Build history of the part. All positions in model axes, mm. A direction names the side the tool comes from. Give positions to 0.01 mm unless a question says otherwise; leave off trailing zeros. Order: outer loops, then holes, each group sorted by start corner. A loop starts at its lowest first (then second) coordinate and runs counter-clockwise, first axis right, second up. Notation, with made-up numbers: M 24.5,54 L 77.5,54 A18 ccw 77.5,77 Z; hole C 69.5,35.25 d7. An arc over 180 degrees is marked long. One line per item, written item: value.
from build123d import *

# Parameters (mm, degrees)
SKETCH1_W           = 25
SKETCH1_H           = 38
BOSS_EXTRUDE1_DEPTH = 1.425
SKETCH2_R           = 2
CUT_EXTRUDE1_DEPTH  = 23.92100565
SKETCH3_R           = 0.8
CUT_EXTRUDE2_DEPTH  = 23.92100565
SKETCH4_W           = 5
SKETCH4_H           = 2.85
BOSS_EXTRUDE2_DEPTH = 2.85
SKETCH5_W           = 8
SKETCH5_H           = 2.9
CUT_EXTRUDE3_DEPTH  = 26.333673243
SKETCH6_W           = 3.5
SKETCH6_H           = 8.95
CUT_EXTRUDE4_DEPTH  = 26.333673243
FILLET1_R           = 5


with BuildPart() as part:
    # Sketch1 → Boss-Extrude1 (new, symmetric)
    with BuildSketch(Plane.XY):
        Rectangle(SKETCH1_W, SKETCH1_H)
    extrude(amount=BOSS_EXTRUDE1_DEPTH, both=True)

    # Sketch2 → Cut-Extrude1 (cut, through all)
    with BuildSketch(Plane.XY.offset(1.425)):
        with Locations((0, -14)):
            Circle(SKETCH2_R)
    extrude(amount=-CUT_EXTRUDE1_DEPTH, mode=Mode.SUBTRACT)

    # Sketch3 → Cut-Extrude2 (cut, through all)
    with BuildSketch(Plane.XY.offset(1.425)):
        with Locations((-4.8, -14)):
            Circle(SKETCH3_R)
        with Locations((4.8, -14)):
            Circle(SKETCH3_R)
    extrude(amount=-CUT_EXTRUDE2_DEPTH, mode=Mode.SUBTRACT)

    # Sketch4 → Boss-Extrude2 (add)
    with BuildSketch(Plane.XY.offset(1.425)):
        with Locations((-4.25, 20.425)):
            Rectangle(SKETCH4_W, SKETCH4_H)
        with Locations((4.25, 20.425)):
            Rectangle(SKETCH4_W, SKETCH4_H)
    extrude(amount=-BOSS_EXTRUDE2_DEPTH)

    # Sketch5 → Cut-Extrude3 (cut, through all)
    with BuildSketch(Plane.XY.offset(1.425)):
        with Locations((0, 14.5)):
            Rectangle(SKETCH5_W, SKETCH5_H)
    extrude(amount=-CUT_EXTRUDE3_DEPTH, mode=Mode.SUBTRACT)

    # Sketch6 → Cut-Extrude4 (cut, through all)
    with BuildSketch(Plane.XY.offset(1.425)):
        with Locations((0, 14.525)):
            Rectangle(SKETCH6_W, SKETCH6_H)
    extrude(amount=-CUT_EXTRUDE4_DEPTH, mode=Mode.SUBTRACT)

    # Fillet1
    fillet1_edges = [part.edges().sort_by_distance(p)[0] for p in [
        (12.5, -19, 0),
        (-12.5, -19, 0),
    ]]
    fillet(fillet1_edges, radius=FILLET1_R)


solid = part.part
1) Saw through at D-D, the plane x = -8.75. Write the cut outline in (y, z) (3 decimals), then the cut area to 3 significant figures.
Check values:
outline: M -18.841,-1.425 L 19,-1.425 L 19,1.425 L -18.841,1.425 Z
area: 108 mm^2
2) Saw through at B-B, the plane z = -1. Write the cut outline in (x, y), then the cut area to 3 significant figures.
Check values:
outline: M -12.5,-14 A5 ccw -7.5,-19 L 7.5,-19 A5 ccw 12.5,-14 L 12.5,19 L 6.75,19 L 6.75,21.85 L 1.75,21.85 L 1.75,15.95 L 4,15.95 L 4,13.05 L 1.75,13.05 L 1.75,10.05 L -1.75,10.05 L -1.75,13.05 L -4,13.05 L -4,15.95 L -1.75,15.95 L -1.75,21.85 L -6.75,21.85 L -6.75,19 L -12.5,19 Z; hole C -4.8,-14 d1.6; hole C 0,-14 d4; hole C 4.8,-14 d1.6
area: 907 mm^2
3) Mould opens along Y. For faces 1 (the face through (-12.5, 2, 0)), 2 (the face through (-3, 15.95, 0)), 3 (the face through (-4, 21.85, 0)) say: released by +Y, released by -Y, zero draft, split by the parting line, or undercut.
Check values:
face 1: zero draft
face 2: undercut
face 3: released by +Y
4) Drill centre lines: probe 1 along Y at (x, z) = (4.8, -0.45); probe 2 along Y at (x, z) = (3.5, -0.8); probe 3 along X at (y, z) = (11, 1.15). Where is each one in solid material? Low to high. Write a range as from..to.
Check values:
probe 1: -19..-14.8, -13.2..21.85
probe 2: -19..13.05, 15.95..21.85
probe 3: -12.5..-1.75, 1.75..12.5
5) Tool access for faces 4 (the face through (6.75, 20, 0)), 5 (the face through (0, 10.05, 0)), 6 (the face through (11.07, -17.5, 0.02)), 7 (the face through (-4, 14, 0)): list every direction of +Z, -Z, +X, -X, +Y, -Y with a clear straight run to the whole face (end or side of a thin tool).
Check values:
face 4: +Z, -Z, +X, +Y
face 5: +Z, -Z, +Y
face 6: +Z, -Z, +X, -Y
face 7: +Z, -Z
6) Saw through at A-A, the plane x = 0. Write the cut outline in (y, z) (3 decimals), then the cut area to 3 significant figures.
Check values:
outline: M -19,-1.425 L -16,-1.425 L -16,1.425 L -19,1.425 Z; M -12,-1.425 L 10.05,-1.425 L 10.05,1.425 L -12,1.425 Z
area: 71.4 mm^2
7) Saw through at C-C, the plane x = -4.8. Write the cut outline in (y, z) (3 decimals).
Check values:
outline: M -19,-1.425 L -14.8,-1.425 L -14.8,1.425 L -19,1.425 Z; M -13.2,-1.425 L 21.85,-1.425 L 21.85,1.425 L -13.2,1.425 Z
